from build123d import *

# Parameters (mm, degrees)
PROFILE_SKETCH_R       = 4.7625
BOSS_EXTRUDE1_DEPTH    = 43.18
PLATE_RELIEF_CUT_REACH = 45.18
PLATE_RELIEF_SKETCH_W  = 6.35
PLATE_RELIEF_SKETCH_H  = 3.175
M3X0_5_TAPPED_HOLE1_D  = 2.5


with BuildPart() as part:
    # Profile Sketch → Boss-Extrude1 (new body)
    with BuildSketch(Plane(origin=(0, 0, 0), x_dir=(1, 0, 0), z_dir=(0, 1, 0))):
        Circle(PROFILE_SKETCH_R)
    extrude(amount=BOSS_EXTRUDE1_DEPTH)

    # Plate Relief Sketch → Plate Relief Cut (cut, up to next)
    with BuildSketch(Plane.XZ, mode=Mode.PRIVATE) as plate_relief_cut_sk1:
        with Locations((-1.315128061, 3.175)):
            Rectangle(PLATE_RELIEF_SKETCH_W, PLATE_RELIEF_SKETCH_H)
    plate_relief_cut_tool1 = extrude(plate_relief_cut_sk1.sketch, amount=-PLATE_RELIEF_CUT_REACH, mode=Mode.PRIVATE) & part.part
    add(plate_relief_cut_tool1.solids().sort_by_distance((-1.315128, 0, 3.175))[0], mode=Mode.SUBTRACT)

    # M3x0.5 Tapped Hole1 (through all)
    with Locations(Plane(origin=(-1.315128061, 34.29, 1.5875), x_dir=(1, 0, 0), z_dir=(0, 0, 1))):
        with Locations((0, 0), (0, -25.4)):
            Hole(M3X0_5_TAPPED_HOLE1_D / 2)


solid = part.part
Could you check a few things on this model? Use its own coordinates, in mm. Coordinates: 2 decimals unless noted, no trailing zeros. Write each loop counter-clockwise with the first axis right and the second up, starting at its lowest first coordinate (ties: lowest second). Pieces come first, ordered by that corner, then holes. Notation, with made-up numbers: (55, 24) - (97, 24) arc R37 cw to (97, 63) - close; hole circle Ø11 at (-32, -12.75). An arc over 180 degrees is marked (long way). Put each result on its own line as item: value. Start each with the question number.
Q1. Thinking about a two-plate mould opening in X: for faces 1 (the cylindrical face through (-0.066, 8.945, -1.632)), 2 (the flat face through (1.86, 21, 3)), 3 (the flat face through (-1, 21, 1.588)), which applies, pulls with the +X half, pulls with the -X half, needs draft (parallel to the pull), parting line crosses it, or undercut?
Q2. Please list where these lines run through material, in increasing order: L1, parallel to X at y = 7.5, z = -0.25; L2, parallel to X at y = 34.5, z = -2.75; L3, parallel to Z at x = 0, y = 15.
Q3. I want a section at A-A on y = 34.29. Write out the boundary of the cut face in (x, z) (1 decimal), plus the area to 3 significant figures.
Q4. I want a section at C-C on x = -4. Write out the boundary of the cut face in (y, z), plus the area to 3 significant figures.
Q5. I'm going to push flat-ended pins straight in: P1, Ø0.8, axis at y = 28, z = 3, coming from the -X side; P2, Ø4, axis at x = -1.32, y = 34.29, coming from the +Z side; P3, Ø2, axis at y = 36, z = 1.5, coming from the -X side. Where does each tip first touch, or does it pass through?
Q6. I want a section at B-B on z = 0. Write out the boundary of the cut face in (x, y).
Q7. I want a section at D-D on y = 12. Write out the boundary of the cut face in (x, z) (1 decimal).
Checks:
1. face 1: undercut
1. face 2: pulls with the -X half
1. face 3: needs draft
2. L1: -4.76 to 4.76
2. L2: -3.89 to -2.55, -0.08 to 3.89
2. L3: -4.76 to 1.59
3. outline: (-4.5, 1.6) arc R4.8 ccw to (-2.6, -4) - (-2.6, 1.6) - close; (-0.1, -4.8) arc R4.8 ccw to (1.9, 4.4) - (1.9, 1.6) - (-0.1, 1.6) - close
3. area: 39.9 mm²
4. outline: (0, -2.58) - (43.18, -2.58) - (43.18, 1.59) - (0, 1.59) - close
4. area: 180 mm²
5. P1: x = 1.86
5. P2: z = 1.59
5. P3: x = -4.74
6. outline: (-4.76, 0) - (4.76, 0) - (4.76, 43.18) - (-4.76, 43.18) - close; hole circle Ø2.5 at (-1.32, 8.89); hole circle Ø2.5 at (-1.32, 34.29)
7. outline: (-4.5, 1.6) arc R4.8 ccw (long way) to (1.9, 4.4) - (1.9, 1.6) - close
